Verification items for the finished model (mm, model axes). Coordinates: 2 decimals unless noted, no trailing zeros. Loops run counter-clockwise (first coordinate to the right, second up) from the corner with the lowest first, then second, coordinate; pieces in that order, holes last. Notation, with made-up numbers: (-28.75, 34.5) -> (23.25, 34.5) arc R23 cw to (23.25, 50.5) -> close; hole circle Ø6 at (52.25, 10). An arc over 180 degrees is marked (long way). Write item = value, one per line.
Autodesk Inventor part; units mm, degrees
ref_plane "YZ Plane" through (0, 0, 0) normal (1, 0, 0) x (0, 1, 0)
ref_plane "XZ Plane" through (0, 0, 0) normal (0, 1, 0) x (-1, 0, 0)
ref_plane "XY Plane" through (0, 0, 0) normal (0, 0, 1) x (1, 0, 0)
sketch "Sketch1" plane through (0, 0, 0) normal (0, 1, 0) x (-1, 0, 0)
  ellipse E0 centre (0, 0) end of major axis (0, -40) minor radius 25
  line L0 (23.4617, 13.8144) -> (8.75, 77.7778)
  line L1 (8.75, 77.7778) -> (-8.75, 77.7778)
  line L2 (-8.75, 77.7778) -> (-23.4617, 13.8144)
  line L3 (23.4617, -13.8144) -> (8.75, -77.7778)
  line L4 (8.75, -77.7778) -> (-8.75, -77.7778)
  line L5 (-8.75, -77.7778) -> (-23.4617, -13.8144)
  point P0 (0, 77.7778)
  point P1 (0, -77.7778)
  dimension "d0" = 25
  dimension "d1" = 40
  dimension "d2" = 77.7778
  dimension "d3" = 77.7778
  dimension "d5" = 17.5
  dimension "d7" = 17.5
extrude "Plate1" add sketch "Sketch1" along normal blind 0.5
equation "\"d5\" = d7"
equation "\"d8\" = Thickness"
equation "\"BendRadius\" = Thickness"
equation "\"BendReliefWidth\" = Thickness"
equation "\"BendReliefDepth\" = 0.5 * Thickness"
equation "\"CornerReliefSize\" = 4 * Thickness"
equation "\"MinimumRemnant\" = 2 * Thickness"
equation "\"TransitionRadius\" = BendRadius"
equation "\"JacobiRadiusSize\" = BendRadius"
equation "\"GapSize\" = Thickness"
properties part number "SLING"
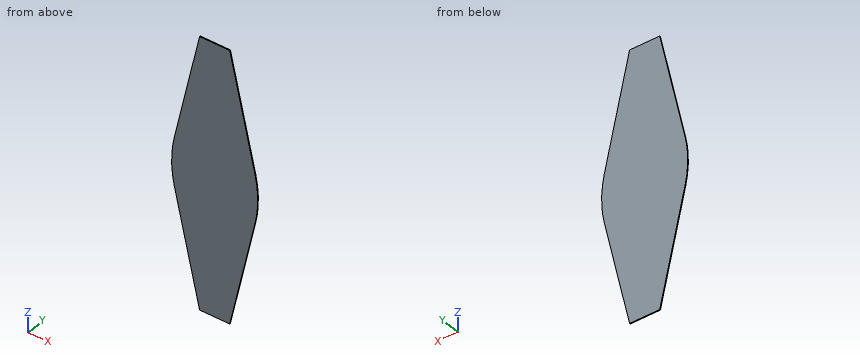
1) Material ranges on line 1 (X direction, y = 0.3, z = 0); line 2 (X direction, y = 0.1, z = -30), recorded low to high.
Ans:
line_1 = -25 to 25
line_2 = -19.74 to 19.74
2) Depth check by flat-ended pin: pin 1 Ø6 at (x, z) = (-2, 22.5) entering from -Y. Enter the tip coordinate at first touch or a pass-through.
Ans:
pin_1 = 0
3) Sectioned sample at B-B, the plane x = 11. Record the cut outline in (y, z), plus the area to 3 significant figures.
Ans:
outline = (0, -68) -> (0.5, -68) -> (0.5, 68) -> (0, 68) -> close
area = 68.0 mm2
4) Sectioned sample at A-A, the plane z = -41. Record the cut outline in (x, y), plus the area to 3 significant figures.
Ans:
outline = (-17.21, 0) -> (17.21, 0) -> (17.21, 0.5) -> (-17.21, 0.5) -> close
area = 17.2 mm2
